Autodesk Inventor part; units mm, degrees
ref_plane "YZ Plane" through (0, 0, 0) normal (1, 0, 0) x (0, 1, 0)
ref_plane "XZ Plane" through (0, 0, 0) normal (0, 1, 0) x (-1, 0, 0)
ref_plane "XY Plane" through (0, 0, 0) normal (0, 0, 1) x (1, 0, 0)
sketch "Sketch1" plane through (0, 0, 0) normal (0, 0, 1) x (1, 0, 0)
  circle A0 centre (0, 0) radius 3.75
  line L0 (10.8, -10.8193) -> (10.8234, 10.804)
  line L1 (-10.8, 10.8274) -> (-10.8234, -10.7959)
  arc A1 (-10.1405, -3.75) -> (-10.1405, 3.75) centre (0, 0) ccw
  line L2 (0, 3.75) -> (-19, 3.75)
  line L3 (0, 3.75) -> (19, 3.75) construction
  line L4 (-19, 3.75) -> (-19, -3.75)
  line L5 (-19, -3.75) -> (0, -3.75)
  point P0 (0, 0)
  dimension "d0" = 19
  dimension "d1" = 180
extrude "Extrusion1" add sketch "Sketch1" along normal blind 8.5 contours A0 L2 A1 L5 | A0 L5 L1 L2 | L1 L5 L4 L2
sketch "Sketch2" plane through (0, 0, 8.5) normal (0, 0, 1) x (1, 0, 0)
  arc A0 (-10.1405, -3.75) -> (-10.1405, 3.75) centre (0, 0) ccw
  circle A1 centre (0, 0) radius 3.75
  circle A2 centre (0, 0) radius 3.75
  line L0 (3.75, 0) -> (3.75, 10.8117)
  line L1 (0, 10.8117) -> (3.75, 10.8117)
  line L2 (-3.75, 0) -> (-3.75, 10.8117)
  line L3 (-3.75, 10.8117) -> (3.75, 10.8117)
  line L4 (0, -10.8117) -> (-3.75, -10.8117)
  line L5 (-3.75, -10.8117) -> (-3.75, 0)
  line L6 (3.75, 0) -> (3.75, -10.8117)
  line L7 (3.75, -10.8117) -> (-3.75, -10.8117)
  point P0 (0, 0)
  point P1 (-3.75, 10.1405)
  point P2 (3.75, 10.1405)
  point P3 (3.75, -10.1405)
  point P4 (-3.75, -10.1405)
extrude "Extrusion2" add sketch "Sketch2" against normal up to surface (8.5 mm away) contours A0 L4 L5 | A0 L6 L7 | L2 L3 A0 | A0 L1 L0
sketch "Sketch3" plane through (-3.75, -10.8117, 8.5) normal (-1, 0, 0) x (0, 0, 1)
  line L0 (0, 0) -> (-8.5, 0)
  line L1 (0, 21.6234) -> (-8.5, 21.6234)
  line L2 (0, 0) -> (0, 0.6712)
  line L3 (0, 0) -> (-6, 0)
  line L4 (0, 0) -> (-8.5, 0)
  line L5 (0, 0) -> (-3, 0)
  line L6 (-3, 0) -> (-3, -6)
  line L7 (-3, 0) -> (3, 0) construction
  circle A0 centre (-3, -3) radius 1.5
  line L8 (0, 21.6234) -> (-3, 21.6234)
  line L9 (-3, 21.6234) -> (-3, 27.6234)
  circle A1 centre (-3, 24.6234) radius 1.5
  circle A2 centre (-3, 24.6234) radius 3
  circle A3 centre (-3, -3) radius 3
  line L10 (0, 0) -> (0, -3)
  line L11 (-8.5, 0) -> (-5.5223, -4.6242)
  line L12 (0, 21.6234) -> (0, 24.6234)
  line L13 (0, 21.6234) -> (-8.5, 21.6234)
  line L14 (-8.5, 21.6234) -> (-5.5223, 26.2476)
  point P0 (-8.5, 10.8117)
  dimension "d6" = 6
  dimension "d7" = 3
  dimension "d8" = 6
  dimension "d9" = 90
  dimension "d10" = 3
  dimension "d11" = 3
  dimension "d12" = 6
  dimension "d13" = 3
extrude "Extrusion3" add sketch "Sketch3" against normal up to surface (7.5 mm away) contours L10 A3 L0 | A3 L11 L0 | A3 L6 A0 | L6 A0 A3 | L1 A2 L12 | A2 L9 A1 | L1 L14 A2 | L9 A1 A2
chamfer "Chamfer1" distance 2 angle 45 2 edges at (-10.1405, -3.75, 4.25) (-10.1405, 3.75, 4.25)
properties part number "NewCameraHolder_3DPrint"
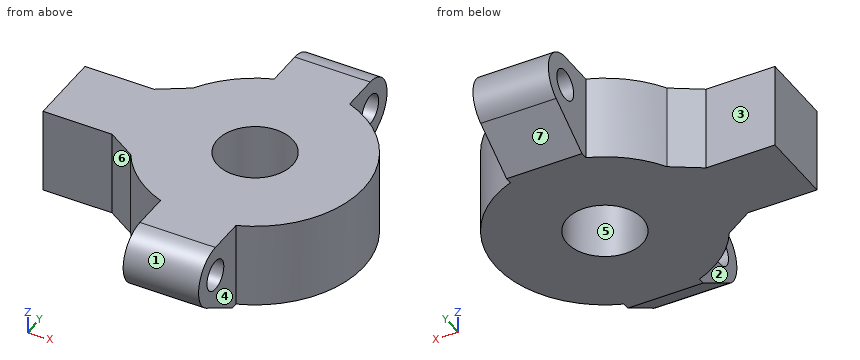
Geometry: final body of the model. Coordinates: model frame, mm. Face numbers are marked on the shaded views. A direction names the side the tool comes from. Coordinates: 2 decimals unless noted, no trailing zeros. Order: outer loops, then holes, each group sorted by start corner. A loop starts at its lowest first (then second) coordinate and runs counter-clockwise, first axis right, second up.
(1) Section query B-B (y = 0). Return the cut outline in (x, z).
(2) Section query C-C (z = 5.5). Return the cut outline in (x, y), plus the area to 3 significant figures.
(3) Section query A-A (x = 0). Return the cut outline in (y, z), plus the area to 3 significant figures.
(4) First-contact query: pin 1 (2 mm diameter, centred on x = -13, y = 0.5, fed in from -Z); pin 2 (3.5 mm diameter, centred on y = 13.81, z = 5.5, fed in from +X); pin 3 (3.5 mm diameter, centred on x = -15, z = 6, fed in from -Y); pin 4 (5 mm diameter, centred on x = -13, z = 7, fed in from +Y). Flat tips, straight axial feed; report the tip coordinate or a pass-through.
(5) Section query D-D (z = 1.75). Return the cut outline in (x, y).
(6) Material intervals for probe 1 along Y at (x, z) = (0, 5.5); probe 2 along X at (y, z) = (0, 3); probe 3 along Y at (x, z) = (-17, 6.75), sorted ascending.
(7) Access query for the marked faces 1, 2, 3 and 4. Directions: +Z, -Z, +X, -X, +Y, -Y. A direction counts if a zero-diameter tool reaches every point of the face in a straight line with its end or side. Return the directions, or none.
(8) Draft query along Y for the marked faces 5, 6 and 7. Return one class per face: pulls with the +Y half, pulls with the -Y half, needs draft (parallel to the pull), parting line crosses it, or undercut.
Solution:
1. outline: (-19, 0) - (-3.75, 0) - (-3.75, 8.5) - (-19, 8.5) - close; (3.75, 0) - (10.81, 0) - (10.81, 8.5) - (3.75, 8.5) - close
2. outline: (-19, -3.75) - (-12.14, -3.75) - (-9.28, -5.55) arc R10.81 ccw to (-3.75, -10.14) - (-3.75, -12.31) - (3.75, -12.31) - (3.75, -10.14) arc R10.81 ccw to (3.75, 10.14) - (3.75, 12.31) - (-3.75, 12.31) - (-3.75, 10.14) arc R10.81 ccw to (-9.28, 5.55) - (-12.14, 3.75) - (-19, 3.75) - close; (-3.75, -16.81) - (3.75, -16.81) - (3.75, -15.31) - (-3.75, -15.31) - close; (-3.75, 15.31) - (3.75, 15.31) - (3.75, 16.81) - (-3.75, 16.81) - close; hole circle Ø7.5 at (0, 0)
2. area: 438 mm2
3. outline: (-15.44, 2.98) - (-10.81, 0) - (-3.75, 0) - (-3.75, 8.5) - (-13.81, 8.5) arc R3 ccw to start; (3.75, 0) - (10.81, 0) - (15.44, 2.98) arc R3 ccw to (13.81, 8.5) - (3.75, 8.5) - close; hole circle Ø3 at (-13.81, 5.5); hole circle Ø3 at (13.81, 5.5)
3. area: 180 mm2
4. pin 1: stops at z = 0
4. pin 2: stops at x = 3.75
4. pin 3: stops at y = -3.75
4. pin 4: stops at y = 4.78
5. outline: (-19, -3.75) - (-12.14, -3.75) - (-9.28, -5.55) arc R10.81 ccw to (-3.75, -10.14) - (-3.75, -13.53) - (3.75, -13.53) - (3.75, -10.14) arc R10.81 ccw to (3.75, 10.14) - (3.75, 13.53) - (-3.75, 13.53) - (-3.75, 10.14) arc R10.81 ccw to (-9.28, 5.55) - (-12.14, 3.75) - (-19, 3.75) - close; hole circle Ø7.5 at (0, 0)
6. probe 1: y = -16.81 to -15.31, -12.31 to -3.75, 3.75 to 12.31, 15.31 to 16.81
6. probe 2: x = -19 to -3.75, 3.75 to 10.81
6. probe 3: y = -3.75 to 3.75
7. face 1: +X, -X, -Y
7. face 2: +Z, -Z, -X, -Y
7. face 3: +Z, -Z, -X, +Y
7. face 4: +Z, -Z, +X, -Y
8. face 5: undercut
8. face 6: pulls with the -Y half
8. face 7: pulls with the +Y half
